from build123d import *

# Parameters (mm, degrees)
PAD_DEPTH       = 26
SKETCH002_W     = 5
SKETCH002_H     = 20
POCKET_DEPTH    = 155.156903
SKETCH004_W     = 10
SKETCH004_H     = 3
POCKET001_DEPTH = 5
SKETCH005_R     = 7.5
POCKET002_DEPTH = 5


with BuildPart() as part:
    # Sketch → Pad (new body)
    with BuildSketch(Plane.XY):
        Polygon((-54, 0), (-28, 0), (-28, -16), (0, -16), (0, -18), (-30, -18), (-30, -2), (-54, -2), align=None)
    pad = extrude(amount=PAD_DEPTH)

    # Sketch002 (on DatumPlane) → Pocket (cut, through all)
    with BuildSketch(Plane(origin=(-30, 0, 0), x_dir=(0, -1, 0), z_dir=(-1, 0, 0))):
        with Locations((4.5, 13)):
            Rectangle(SKETCH002_W, SKETCH002_H)
    pocket = extrude(amount=-POCKET_DEPTH, mode=Mode.SUBTRACT)

    # Sketch004 (on DatumPlane) → Pocket001 (cut)
    with BuildSketch(Plane.XZ.offset(2)):
        with Locations((-41, 24.53954)):
            Rectangle(SKETCH004_W, SKETCH004_H)
        with Locations((-41, 1.5)):
            Rectangle(SKETCH004_W, SKETCH004_H)
    pocket001 = extrude(amount=-POCKET001_DEPTH, mode=Mode.SUBTRACT)

    # Sketch005 (on DatumPlane) → Pocket002 (cut)
    with BuildSketch(Plane.XZ.offset(18)):
        with Locations((-0.570245, 13)):
            Circle(SKETCH005_R)
    extrude(amount=-POCKET002_DEPTH, mode=Mode.SUBTRACT)

    # Mirrored: Pad across Sketch V_Axis
    add(pad.mirror(Plane(origin=(0, 0, 0), x_dir=(0, 0, 1), z_dir=(1, 0, 0))))

    # Mirrored001: Pocket across YZ
    add(pocket.mirror(Plane.YZ), mode=Mode.SUBTRACT)

    # Mirrored002: Pocket001 across Sketch004 V_Axis
    add(pocket001.mirror(Plane(origin=(0, -2, 0), x_dir=(0, -1, 0), z_dir=(1, 0, 0))), mode=Mode.SUBTRACT)


solid = part.part
Geometry: final body of the model. Coordinates: model frame, mm. A direction names the side the tool comes from. Coordinates: 2 decimals unless noted, no trailing zeros. Order: outer loops, then holes, each group sorted by start corner. A loop starts at its lowest first (then second) coordinate and runs counter-clockwise, first axis right, second up.
(1) Section query D-D (x = -4). Return the cut outline in (y, z), plus the area to 3 significant figures.
(2) Draft query along X for faces 1 (the face through (-41, -1, 3)), 2 (the face through (29, -4, 23)), 3 (the face through (41, -1, 3)), 4 (the face through (-54, -1, 13)). Return one class per face: pulls with the +X half, pulls with the -X half, needs draft (parallel to the pull), parting line crosses it, or undercut.
(3) Material intervals for probe 1 along X at (y, z) = (-1.25, 1.25); probe 2 along X at (y, z) = (-15, 17.25); probe 3 along Y at (x, z) = (25.5, 8.25), sorted ascending.
(4) First-contact query: pin 1 (1 mm diameter, centred on y = -15, z = 16.5, fed in from -X); pin 2 (1.5 mm diameter, centred on y = -11, z = 7, fed in from +X); pin 3 (13 mm diameter, centred on x = 12, z = 17, fed in from +Y). Flat tips, straight axial feed; report the tip coordinate or a pass-through.
(5) Section query A-A (z = 21.5). Return the cut outline in (x, y).
(6) Section query C-C (z = 13). Return the cut outline in (x, y).
(7) Section query B-B (y = -9). Return the cut outline in (x, z), plus the area to 3 significant figures.
(8) Access query for faces 5 (the face through (-30, -12, 13)), 6 (the face through (30, -12, 13)), 7 (the face through (-36, -1, 1)), 8 (the face through (-36, -1, 24)), 9 (the face through (29, -7, 13)). Directions: +Z, -Z, +X, -X, +Y, -Y. A direction counts if a zero-diameter tool reaches every point of the face in a straight line with its end or side. Return the directions, or none.
Solution:
1. outline: (-18, 0) - (-16, 0) - (-16, 6.33) - (-18, 6.33) - close; (-18, 19.67) - (-16, 19.67) - (-16, 26) - (-18, 26) - close
1. area: 25.3 mm2
2. face 1: undercut
2. face 2: needs draft
2. face 3: undercut
2. face 4: pulls with the -X half
3. probe 1: x = -54 to -46, -36 to -28, 28 to 36, 46 to 54
3. probe 2: x = -30 to -28, 28 to 30
3. probe 3: y = -18 to -16
4. pin 1: stops at x = -30
4. pin 2: stops at x = 30
4. pin 3: stops at y = -16
5. outline: (-54, -2) - (-28, -2) - (-28, 0) - (-54, 0) - close; (-30, -18) - (30, -18) - (30, -7) - (28, -7) - (28, -16) - (-28, -16) - (-28, -7) - (-30, -7) - close; (28, -2) - (54, -2) - (54, 0) - (28, 0) - close
6. outline: (-54, -2) - (-28, -2) - (-28, 0) - (-54, 0) - close; (-30, -18) - (-8.07, -18) - (-8.07, -16) - (-28, -16) - (-28, -7) - (-30, -7) - close; (0, -18) - (30, -18) - (30, -7) - (28, -7) - (28, -16) - (0, -16) - close; (28, -2) - (54, -2) - (54, 0) - (28, 0) - close
7. outline: (-30, 0) - (-28, 0) - (-28, 26) - (-30, 26) - close; (28, 0) - (30, 0) - (30, 26) - (28, 26) - close
7. area: 104 mm2
8. face 5: +Z, -Z, -X, -Y
8. face 6: +Z, -Z, +X, -Y
8. face 7: -Z, +Y, -Y
8. face 8: +Z, +Y, -Y
8. face 9: +X, -X
